Check sheet for the modelled part. Datum: model origin and axes. Units: mm. A direction names the side the tool comes from. Coordinates: 2 decimals unless noted, no trailing zeros. Loops run counter-clockwise (first coordinate to the right, second up) from the corner with the lowest first, then second, coordinate; pieces in that order, holes last. Notation, with made-up numbers: (-14, -27.5) - (5, -27.5) arc R33 cw to (5, 1.5) - close; hole circle Ø6 at (73, 4.25). An arc over 180 degrees is marked (long way). Use a Markdown table: item, result. Add a question column.
1) Sectioned sample at C-C, the plane y = 0. Enter the section's corners in (x, z).
2) Tool access check on faces 1 (the flat face through (16, 0, 4)), 2 (the flat face through (-7.5, 9.5, 2.5)), 3 (the flat face through (16, -4.8, 2)), 4 (the flat face through (16, 4.8, 2)), 5 (the flat face through (7, 0, 0)). Record the directions out of +Z, -Z, +X, -X, +Y, -Y that give a thin tool (end or side, any length) a straight path to the whole face; none if there is none.
3) Go/stop test with flat-tipped pins: P1, Ø3, axis at x = 19.5, z = 2.5, coming from the -Y side; P2, Ø10.5, axis at x = 17.5, y = -1.5, coming from the +Z side; P3, Ø3, axis at x = 8, z = 4.5, coming from the +Y side. Record where each tip stops, or that it passes through.
4) Thickness scan on line 1 (X direction, y = 0, z = 1.2); line 2 (Y direction, x = 25, z = 1.5); line 3 (X direction, y = -5, z = 4.5). Record the ranges inside material, lowest first.
5) Draft check along Y on faces 6 (the flat face through (-3, -10, 2)), 7 (the flat face through (-3, 10, 2)), 8 (the cylindrical face through (23.6, 1.284, 1.972)). Enter one of: pulls with the +Y half, pulls with the -Y half, needs draft (parallel to the pull), parting line crosses it, or undercut.
6) Sectioned sample at B-B, the plane x = 25. Enter the section's corners in (y, z), then the cut area to 3 significant figures.
7) Sectioned sample at D-D, the plane y = -2.25. Enter the section's corners in (x, z), then the cut area to 3 significant figures.
8) Sectioned sample at A-A, the plane z = 3.65. Enter the section's corners in (x, y), then the cut area to 3 significant figures.
from build123d import *

# Parameters (mm, degrees)
CYLINDER025_R     = 1.9
CYLINDER025_DEPTH = 5
BOX018_W          = 30
BOX018_H          = 9.6
BOX018_DEPTH      = 4
BOX019_W          = 10
BOX019_H          = 20
BOX019_DEPTH      = 5
CHAMFER009_SIZE   = 1


with BuildPart() as cylinder025:
    # Cylinder025 → Cylinder025 (new body)
    with BuildSketch(Plane(origin=(25, 0, 0), x_dir=(1, 0, 0), z_dir=(0, 0, 1))):
        Circle(CYLINDER025_R)
    extrude(amount=CYLINDER025_DEPTH)


with BuildPart() as cut002008023012009006003002006_body:
    # Box018 → Box018 (new body)
    with BuildSketch(Plane(origin=(0, -4.8, 0), x_dir=(1, 0, 0), z_dir=(0, 0, 1))):
        with Locations((15, 4.8)):
            Rectangle(BOX018_W, BOX018_H)
    extrude(amount=BOX018_DEPTH)

    # Cut002008023012009006003002006002006002004004002: cut Cylinder025
    add(cylinder025.part, mode=Mode.SUBTRACT)


with BuildPart() as fusion001001001011002004:
    # Box019 → Box019 (new body)
    with BuildSketch(Plane(origin=(-8, -10, 0), x_dir=(1, 0, 0), z_dir=(0, 0, 1))):
        with Locations((5, 10)):
            Rectangle(BOX019_W, BOX019_H)
    extrude(amount=BOX019_DEPTH)

    # Chamfer009
    chamfer009_edges = [fusion001001001011002004.edges().sort_by_distance(p)[0] for p in [
        (-8, -10, 2.5),
        (-8, 10, 2.5),
    ]]
    chamfer(chamfer009_edges, length=CHAMFER009_SIZE)

    # Fusion001001001011002004: union Cut002008023012009006003002006 body
    add(cut002008023012009006003002006_body.part)


solid = fusion001001001011002004.part
Solved:
| question | item | result |
|---|---|---|
| 1 | outline | (-8, 0) - (23.1, 0) - (23.1, 4) - (2, 4) - (2, 5) - (-8, 5) - close; (26.9, 0) - (30, 0) - (30, 4) - (26.9, 4) - close |
| 2 | face 1 | +Z, +X, +Y, -Y |
| 2 | face 2 | +Z, -Z, -X, +Y |
| 2 | face 3 | +Z, -Z, +X, -Y |
| 2 | face 4 | +Z, -Z, +X, +Y |
| 2 | face 5 | -Z, +X, -X, +Y, -Y |
| 3 | P1 | stops at y = -4.8 |
| 3 | P2 | stops at z = 4 |
| 3 | P3 | stops at y = 4.8 |
| 4 | line 1 | x = -8 to 23.1, 26.9 to 30 |
| 4 | line 2 | y = -4.8 to -1.9, 1.9 to 4.8 |
| 4 | line 3 | x = -8 to 2 |
| 5 | face 6 | pulls with the -Y half |
| 5 | face 7 | pulls with the +Y half |
| 5 | face 8 | undercut |
| 6 | outline | (-4.8, 0) - (-1.9, 0) - (-1.9, 4) - (-4.8, 4) - close; (1.9, 0) - (4.8, 0) - (4.8, 4) - (1.9, 4) - close |
| 6 | area | 23.2 mm2 |
| 7 | outline | (-8, 0) - (30, 0) - (30, 4) - (2, 4) - (2, 5) - (-8, 5) - close |
| 7 | area | 162 mm2 |
| 8 | outline | (-8, -9) - (-7, -10) - (2, -10) - (2, -4.8) - (30, -4.8) - (30, 4.8) - (2, 4.8) - (2, 10) - (-7, 10) - (-8, 9) - close; hole circle Ø3.8 at (25, 0) |
| 8 | area | 456 mm2 |
